Verification items for the finished model (mm, model axes). Face numbers are marked on the shaded views. A direction names the side the tool comes from. Give positions to 0.01 mm unless a question says otherwise; leave off trailing zeros. Write each loop counter-clockwise with the first axis right and the second up, starting at its lowest first coordinate (ties: lowest second). Pieces come first, ordered by that corner, then holes. Notation, with made-up numbers: M 16,40 L 59,40 A21 cw 59,69 Z; hole C -38,-35 d9. An arc over 180 degrees is marked long. Answer as a JSON object with one key per item and string values.
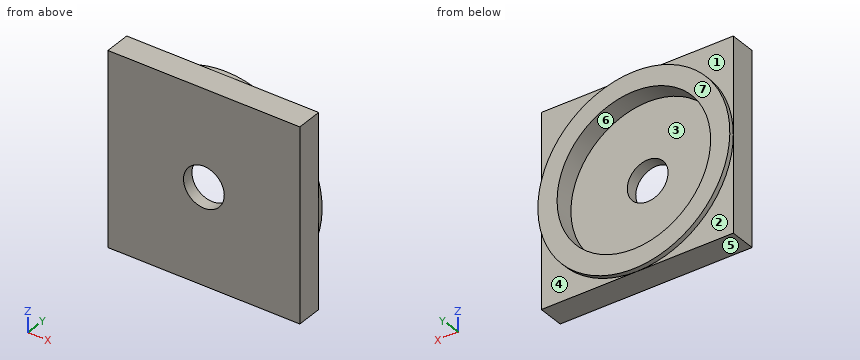
```python
from build123d import *

# Parameters (mm, degrees)
SKETCH2_W           = 63.5
SKETCH2_H           = 63.5
BOSS_EXTRUDE1_DEPTH = 8.636
SKETCH3_R           = 31.75
BOSS_EXTRUDE2_DEPTH = 1.5875
SKETCH4_R           = 25.4
CUT_EXTRUDE1_DEPTH  = 6.35
SKETCH5_R           = 6.74624
CUT_EXTRUDE3_DEPTH  = 46.348070521


with BuildPart() as part:
    # Sketch2 → Boss-Extrude1 (new body)
    with BuildSketch(Plane(origin=(0, 0, 0), x_dir=(1, 0, 0), z_dir=(0, 1, 0))):
        Rectangle(SKETCH2_W, SKETCH2_H)
    extrude(amount=-BOSS_EXTRUDE1_DEPTH)

    # Sketch3 → Boss-Extrude2 (add)
    with BuildSketch(Plane(origin=(0, 0, 0), x_dir=(1, 0, 0), z_dir=(0, 1, 0))):
        with Locations(Location((0, 0, 0), (0, 0, 270))):
            Circle(SKETCH3_R)
    extrude(amount=BOSS_EXTRUDE2_DEPTH)

    # Sketch4 → Cut-Extrude1 (cut)
    with BuildSketch(Plane(origin=(0, 1.5875, 0), x_dir=(1, 0, 0), z_dir=(0, 1, 0))):
        with Locations(Location((0, 0, 0), (0, 0, 270))):
            Circle(SKETCH4_R)
    extrude(amount=-CUT_EXTRUDE1_DEPTH, mode=Mode.SUBTRACT)

    # Sketch5 → Cut-Extrude3 (cut, through all)
    with BuildSketch(Plane(origin=(0, -4.7625, 0), x_dir=(1, 0, 0), z_dir=(0, 1, 0))):
        with Locations(Location((0, 0, 0), (0, 0, 270))):
            Circle(SKETCH5_R)
    extrude(amount=-CUT_EXTRUDE3_DEPTH, mode=Mode.SUBTRACT)


solid = part.part
```
1) Section check C-C on y = -6. Record the boundary of the cut face in (x, z), and give its area (3 significant figures).
Completed:
{"outline": "M -31.75,-31.75 L 31.75,-31.75 L 31.75,31.75 L -31.75,31.75 Z; hole C 0,0 d13.49", "area": "3,890 mm2"}
2) Section check D-D on z = -17. Record the boundary of the cut face in (x, y), and give its area (3 significant figures).
Completed:
{"outline": "M -31.75,-8.64 L 31.75,-8.64 L 31.75,0 L 26.82,0 L 26.82,1.59 L 18.87,1.59 L 18.87,-4.76 L -18.87,-4.76 L -18.87,1.59 L -26.82,1.59 L -26.82,0 L -31.75,0 Z", "area": "394 mm2"}
3) Section check B-B on z = -3. Record the boundary of the cut face in (x, y).
Completed:
{"outline": "M -31.75,-8.64 L -6.04,-8.64 L -6.04,-4.76 L -25.22,-4.76 L -25.22,1.59 L -31.61,1.59 L -31.61,0 L -31.75,0 Z; M 6.04,-8.64 L 31.75,-8.64 L 31.75,0 L 31.61,0 L 31.61,1.59 L 25.22,1.59 L 25.22,-4.76 L 6.04,-4.76 Z"}
4) Release check for a two-part mould opening along Z. For the marked faces 5, 6 and 7 record: pulls with the +Z half, pulls with the -Z half, needs draft (parallel to the pull), parting line crosses it, or undercut.
Completed:
{"face 5": "pulls with the -Z half", "face 6": "undercut", "face 7": "needs draft"}
5) Access from +Z, -Z, +X, -X, +Y, -Y to the whole of each face (thin tool, end or side, straight path). Record for the marked faces 1, 2, 3 and 4.
Completed:
{"face 1": "+Z, -X, +Y", "face 2": "-Z, -X, +Y", "face 3": "+Y", "face 4": "-Z, +X, +Y"}
6) Section check A-A on x = -3. Record the boundary of the cut face in (y, z).
Completed:
{"outline": "M -8.64,-31.75 L 0,-31.75 L 0,-31.61 L 1.59,-31.61 L 1.59,-25.22 L -4.76,-25.22 L -4.76,-6.04 L -8.64,-6.04 Z; M -8.64,6.04 L -4.76,6.04 L -4.76,25.22 L 1.59,25.22 L 1.59,31.61 L 0,31.61 L 0,31.75 L -8.64,31.75 Z"}
7) Go/stop test with a flat-tipped pin: pin 1 (15.5 mm diameter, centred on x = 0, z = 0, fed in from +Y). Record where the tip stops, or that it passes through.
Completed:
{"pin 1": "stops at y = -4.76"}
8) Thickness scan on L1, parallel to X at y = -5.8, z = 0; L2, parallel to X at y = -2, z = 0; L3, parallel to Y at x = -2.5, z = -9. Record the ranges inside material, lowest first.
Completed:
{"L1": "x = -31.75 to -6.75, 6.75 to 31.75", "L2": "x = -31.75 to -25.4, 25.4 to 31.75", "L3": "y = -8.64 to -4.76"}
